```python
from build123d import *

# Parameters (mm, degrees)
ESQUISSE1_R        = 1.5
BOSS_EXTRU_1_DEPTH = 4


with BuildPart() as part:
    # Esquisse1 → Boss.-Extru.1 (new body)
    with BuildSketch(Plane.XY):
        with BuildLine():
            Line((0, 2.5), (35, 2.5))
            ThreePointArc((35, 2.5), (37.5, 0), (35, -2.5))
            Line((35, -2.5), (0, -2.5))
            ThreePointArc((0, -2.5), (-2.5, 0), (0, 2.5))
        make_face()
        Circle(ESQUISSE1_R, mode=Mode.SUBTRACT)
        with Locations((35, 0)):
            Circle(ESQUISSE1_R, mode=Mode.SUBTRACT)
        with BuildLine():
            Line((4.5, 1), (30.5, 1))
            ThreePointArc((30.5, 1), (31.5, 0), (30.5, -1))
            Line((30.5, -1), (4.5, -1))
            ThreePointArc((4.5, -1), (3.5, 0), (4.5, 1))
        make_face(mode=Mode.SUBTRACT)
    extrude(amount=BOSS_EXTRU_1_DEPTH)


solid = part.part
```
Geometry: final body of the model. Coordinates: model frame, mm. A direction names the side the tool comes from. Round coordinates to 2 decimals unless told otherwise and drop trailing zeros. Order: outer loops, then holes, each group sorted by start corner. A loop starts at its lowest first (then second) coordinate and runs counter-clockwise, first axis right, second up. Notation, with made-up numbers: M 12.5,-12.75 L 48.5,-12.75 A29 ccw 48.5,15.25 Z; hole C 38,67.5 d4. An arc over 180 degrees is marked long. Use one line per item in the form item = value. Start each with the question number.
Q1. Material intervals for line 1 (X direction, y = 0.05, z = 3.3); line 2 (Y direction, x = 14.5, z = 0.75); line 3 (Y direction, x = 0, z = 0.9), sorted ascending. Write a range as [from, to].
Q2. Cut plane B-B (x = 27). Return loops of the section in (y, z).
Q3. Access query for faces 4 (the face through (17, 1, 2)), 5 (the face through (18, 2, 4)). Directions: +Z, -Z, +X, -X, +Y, -Y. A direction counts if a zero-diameter tool reaches every point of the face in a straight line with its end or side. Return the directions, or none.
Q4. Cut plane D-D (y = 1.95). Return loops of the section in (x, z).
Q5. Mould query, pull axis X, two halves, no side actions, for faces 1 (the face through (17, 2.5, 2)), 2 (the face through (18, -1, 2)), 3 (the face through (-2.5, -0.1, 2)). Classes: +X half, -X half, draft (parallel to the pull), parting line (faces both ways), or undercut.
Q6. Cut plane C-C (z = 3). Return loops of the section in (x, y), and give its area (3 significant figures).
Q7. Cut plane A-A (y = 0). Return loops of the section in (x, z).
Q8. Pin query (flat end, axial travel): pin 1 Ø1.5 at (y, z) = (1.5, 1) entering from -X. Return the tip coordinate at first contact, or that it passes through.
Geometry results:
q1.line_1 = [-2.5, -1.5], [1.5, 3.5], [31.5, 33.5], [36.5, 37.5]
q1.line_2 = [-2.5, -1], [1, 2.5]
q1.line_3 = [-2.5, -1.5], [1.5, 2.5]
q2.outline = M -2.5,0 L -1,0 L -1,4 L -2.5,4 Z; M 1,0 L 2.5,0 L 2.5,4 L 1,4 Z
q3.face_4 = +Z, -Z
q3.face_5 = +Z, +X, -X, +Y, -Y
q4.outline = M -1.56,0 L 36.56,0 L 36.56,4 L -1.56,4 Z
q5.face_1 = draft
q5.face_2 = undercut
q5.face_3 = -X half
q6.outline = M 0,-2.5 L 35,-2.5 A2.5 ccw 35,2.5 L 0,2.5 A2.5 ccw Z; hole C 0,0 d3; hole M 4.5,-1 L 30.5,-1 A1 ccw 30.5,1 L 4.5,1 A1 ccw Z; hole C 35,0 d3
q6.area = 125 mm^2
q7.outline = M -2.5,0 L -1.5,0 L -1.5,4 L -2.5,4 Z; M 1.5,0 L 3.5,0 L 3.5,4 L 1.5,4 Z; M 31.5,0 L 33.5,0 L 33.5,4 L 31.5,4 Z; M 36.5,0 L 37.5,0 L 37.5,4 L 36.5,4 Z
q8.pin_1 = -2.38
